CAD build for the part. Positions are in the model's coordinates, mm. Face numbers are marked on the shaded views. A direction names the side the tool comes from. Coordinates: 2 decimals unless noted, no trailing zeros. Loops run counter-clockwise (first coordinate to the right, second up) from the corner with the lowest first, then second, coordinate; pieces in that order, holes last.
1) Which spindle directions (+Z, -Z, +X, -X, +Y, -Y) get a long thin tool onto all of the face, cutting with end or side? Do the marked faces 4, 5, 6, 7 and 8. Say none if no direction does.
2) Wall check: line 1 along Z through (x, y) = (27.7, 7.7); line 2 along Y through (x, z) = (28.6, 0); line 3 along X through (y, z) = (1, -0.1). Give the ranges that are in metal, low to high.
3) Saw through at B-B, the plane x = 23.5. Write the cut outline in (y, z).
4) Saw through at A-A, the plane z = 2.6. Write the cut outline in (x, y), and give its area (3 significant figures).
5) Pin check, flat tips, straight feed: pin 1 Ø1.5 at (y, z) = (6.5, 2.5) entering from -X; pin 2 Ø2 at (x, z) = (15, 0.5) entering from +Y; pin 3 Ø1 at (y, z) = (4.5, 2) entering from +X. Stop position of each tip, or through.
6) Saw through at C-C, the plane x = 12. Write the cut outline in (y, z), and give its area (3 significant figures).
7) Two-plate mould, pull along X, no slides. Class the marked faces 1, 2 and 3: +X half, -X half, draft (parallel to the pull), parting line (faces both ways), or undercut.
```python
from build123d import *

# Parameters (mm, degrees)
EXTRUSION1_DEPTH                  = 3
ESQUISSE2_W                       = 3
ESQUISSE2_H                       = 3
EXTRUSION2_DEPTH                  = 1.2
ESQUISSE3_W                       = 3
ESQUISSE3_H                       = 3
EXTRUSION3_DEPTH                  = 1.2
DIAM_TRE_DU_PER_AGE_4_0_4_1_D     = 4
DIAM_TRE_DU_PER_AGE_4_0_4_1_DEPTH = 3
DIAM_TRE_DU_PER_AGE_4_0_4_1_TIP   = 1.201721238
ESQUISSE6_R                       = 1.525615423
EXTRUSION4_DEPTH                  = 0.1


with BuildPart() as part:
    # Esquisse1 → Extrusion1 (new body, symmetric)
    with BuildSketch(Plane.XY):
        with BuildLine():
            Line((0, 0), (0, 1.5))
            ThreePointArc((0, 1.5), (3.484063784, 6.45860997), (8, 10.5))
            Line((8, 10.5), (30, 10.5))
            Line((30, 10.5), (30, 1))
            Line((30, 1), (27, 1))
            Line((27, 1), (27, 3.5))
            Line((27, 3.5), (14, 3.5))
            Line((14, 3.5), (14, 0))
            Line((14, 0), (0, 0))
        make_face()
    extrude(amount=EXTRUSION1_DEPTH, both=True)

    # Esquisse2 → Extrusion2 (add)
    with BuildSketch(Plane(origin=(0, 10.5, 0), x_dir=(1, 0, 0), z_dir=(0, 1, 0))):
        with Locations((28.5, 0)):
            Rectangle(ESQUISSE2_W, ESQUISSE2_H)
    extrude(amount=EXTRUSION2_DEPTH)

    # Esquisse3 → Extrusion3 (add)
    with BuildSketch(Plane.XZ.offset(-1)):
        with Locations((28.5, 0)):
            Rectangle(ESQUISSE3_W, ESQUISSE3_H)
    extrude(amount=EXTRUSION3_DEPTH)

    # Diamètre du perçage Ø4.0 (4)1
    with Locations(Plane(origin=(30, 0, 0), x_dir=(0, 0, -1), z_dir=(1, 0, 0))):
        with Locations((0, 7.7)):
            Hole(DIAM_TRE_DU_PER_AGE_4_0_4_1_D / 2, depth=DIAM_TRE_DU_PER_AGE_4_0_4_1_DEPTH)
            with Locations((0, 0, -(DIAM_TRE_DU_PER_AGE_4_0_4_1_DEPTH + DIAM_TRE_DU_PER_AGE_4_0_4_1_TIP / 2))):  # 118° drill point
                Cone(0, DIAM_TRE_DU_PER_AGE_4_0_4_1_D / 2, DIAM_TRE_DU_PER_AGE_4_0_4_1_TIP, mode=Mode.SUBTRACT)

    # Esquisse6 → Extrusion4 (add)
    with BuildSketch(Plane.XZ.offset(0.2)):
        with Locations((28.525615423, 0)):
            Circle(ESQUISSE6_R)
    extrude(amount=EXTRUSION4_DEPTH)


solid = part.part
```
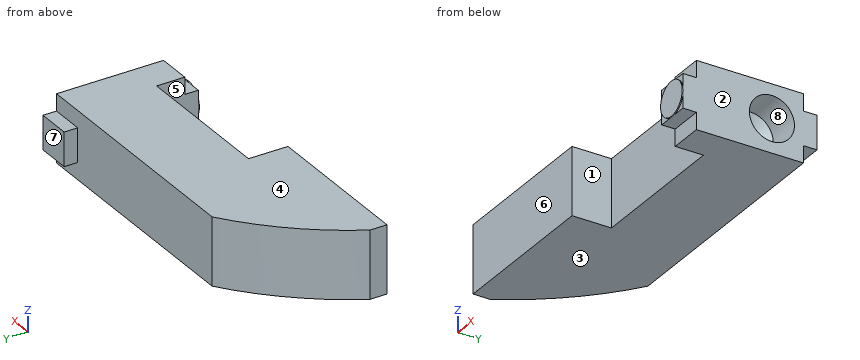
Data:
1. face 4: +Z, +X, -X, +Y, -Y
1. face 5: +Z, -Z, -Y
1. face 6: +Z, -Z, -X, -Y
1. face 7: +Z, -Z, +X, -X, +Y
1. face 8: +X
2. line 1: z = -3 to -2, 2 to 3
2. line 2: y = -0.3 to 5.7, 9.7 to 11.7
2. line 3: x = 0 to 14, 27 to 30
3. outline: (3.5, -3) - (10.5, -3) - (10.5, 3) - (3.5, 3) - close
4. outline: (0, 0) - (14, 0) - (14, 3.5) - (27, 3.5) - (27, 1) - (30, 1) - (30, 10.5) - (8, 10.5) arc R26.6 ccw to (0, 1.5) - close
4. area: 236 mm2
5. pin 1: stops at x = 2.88
5. pin 2: stops at y = 10.5
5. pin 3: stops at x = 30
6. outline: (0, -3) - (10.5, -3) - (10.5, 3) - (0, 3) - close
6. area: 63.0 mm2
7. face 1: undercut
7. face 2: +X half
7. face 3: draft
